```python
from build123d import *

# Parameters (mm, degrees)
F0_W     = 55
F0_H     = 68.072
F1_DEPTH = 12.7
F2_R     = 3.556
F3_DEPTH = 6
F4_DEPTH = 12.7
F5_W     = 55
F5_H     = 10.8541566
F6_DEPTH = 19


with BuildPart() as f1:
    # F0 (on Top) → F1 (new body)
    with BuildSketch(Plane.XY):
        with Locations((-0.5289506033, -7.0382300764)):
            Rectangle(F0_W, F0_H)
    extrude(amount=F1_DEPTH)

    # F2 (on face) → F3 (cut)
    with BuildSketch(Plane.XY.offset(12.7)):
        Polygon((-14.4, -22.3120522499), (-17.9, -28.3742300764), (-14.4, -34.4364079029), (-7.4, -34.4364079029), (-3.9, -28.3742300764), (-7.4, -22.3120522499), align=None)
        with Locations((-10.9, -28.3742300764)):
            Circle(F2_R, mode=Mode.SUBTRACT)
        Polygon((14.456, -34.4364079029), (17.956, -28.3742300764), (14.456, -22.3120522499), (7.456, -22.3120522499), (3.956, -28.3742300764), (7.456, -34.4364079029), align=None)
        with Locations((10.956, -28.3742300764)):
            Circle(F2_R, mode=Mode.SUBTRACT)
    extrude(amount=-F3_DEPTH, mode=Mode.SUBTRACT)

    # F4 (cut, through all): faces of the model
    f4_faces = [f1.faces().sort_by_distance(p)[0] for p in [
        (-10.9, -28.3742300764, 12.7),
        (10.956, -28.3742300764, 12.7),
    ]]
    extrude(f4_faces, amount=-F4_DEPTH, mode=Mode.SUBTRACT)

    # F5 (on face) → F6 (join)
    with BuildSketch(Plane.XY.offset(12.7)):
        with Locations((-0.5289506033, 21.5706916236)):
            Rectangle(F5_W, F5_H)
    extrude(amount=F6_DEPTH)


solid = f1.part
```
The listing builds one solid part. Answer for the finished solid, in the listing's coordinates (mm). A direction names the side the tool comes from. Give positions to 0.01 mm unless a question says otherwise; leave off trailing zeros. Loops run counter-clockwise (first coordinate to the right, second up) from the corner with the lowest first, then second, coordinate; pieces in that order, holes last. Notation, with made-up numbers: (10, 85) - (37, 85) arc R25 cw to (37, 105) - close; hole circle Ø6 at (89, 45). An arc over 180 degrees is marked (long way). Return JSON: item names as keys, results as strings. Group by question number.
1. Given pin 1 Ø2 at (x, z) = (13, 22) entering from -Y; pin 2 Ø13.5 at (x, y) = (-10.5, -25.5) entering from +Z; pin 3 Ø6.5 at (x, y) = (10.96, -28.37) entering from +Z; pin 4 Ø8 at (x, y) = (-10.9, -28.37) entering from +Z, each flat-ended and moving along its own axis, determine where each tip first touches the part or whether it passes through.
2. Find section D-D (z = 25.5). Write down the section's boundary in (x, y), then the cut area to 3 significant figures.
3. Find section C-C (x = 22.5). Write down the section's boundary in (y, z), then the cut area to 3 significant figures.
4. Determine the mould class of faces 4 (the flat face through (-1, 16.144, 22)), 5 (the flat face through (-28.029, -8, 9)), 6 (the cylindrical face through (7.403, -28.218, 3.397)), 7 (the flat face through (26.971, -8, 9)) for opening direction X: pulls with the +X half, pulls with the -X half, needs draft (parallel to the pull), parting line crosses it, or undercut.
5. Find section B-B (z = 4). Write down the section's boundary in (x, y).
6. Find section A-A (x = -10.9). Write down the section's boundary in (y, z), then the cut area to 3 significant figures.
7. Which of the six approach directions +Z, -Z, +X, -X, +Y, -Y give full straight-line access (tool end or side, diameter ignored) to faces 1 (the flat face through (-16.125, -25.301, 9.742)), 2 (the flat face through (-1, -12, 12.7)), 3 (the flat face through (-1, 26.998, 16))?
8. Straight lines are drawn through the part: line 1 (Y direction, x = -13.5, z = 12.5); line 2 (Y direction, x = -10.9, z = 4); line 3 (X direction, y = -28, z = 3.5). For each, find the intervals that lie inside material, in ascending order. Write a range as [from, to].
Verdict:
{
 "1": {"pin 1": "stops at y = 16.14", "pin 2": "stops at z = 12.7", "pin 3": "passes through", "pin 4": "stops at z = 6.7"},
 "2": {"outline": "(-28.03, 16.14) - (26.97, 16.14) - (26.97, 27) - (-28.03, 27) - close", "area": "597 mm^2"},
 "3": {"outline": "(-41.07, 0) - (27, 0) - (27, 31.7) - (16.14, 31.7) - (16.14, 12.7) - (-41.07, 12.7) - close", "area": "1,070 mm^2"},
 "4": {"face 4": "needs draft", "face 5": "pulls with the -X half", "face 6": "undercut", "face 7": "pulls with the +X half"},
 "5": {"outline": "(-28.03, -41.07) - (26.97, -41.07) - (26.97, 27) - (-28.03, 27) - close; hole circle Ø7.11 at (-10.9, -28.37); hole circle Ø7.11 at (10.96, -28.37)"},
 "6": {"outline": "(-41.07, 0) - (-31.93, 0) - (-31.93, 6.7) - (-34.44, 6.7) - (-34.44, 12.7) - (-41.07, 12.7) - close; (-24.82, 0) - (27, 0) - (27, 31.7) - (16.14, 31.7) - (16.14, 12.7) - (-22.31, 12.7) - (-22.31, 6.7) - (-24.82, 6.7) - close", "area": "950 mm^2"},
 "7": {"face 1": "+Z", "face 2": "+Z, +X, -X, -Y", "face 3": "+Z, -Z, +X, -X, +Y"},
 "8": {"line 1": "y = [-41.07, -34.44], [-22.31, 27]", "line 2": "y = [-41.07, -31.93], [-24.82, 27]", "line 3": "x = [-28.03, -14.44], [-7.36, 7.42], [14.49, 26.97]"}
}
